Check sheet for the drawn part. Datum: minimum x, y, z corner. Units: mm. A direction names the side the tool comes from. Round coordinates to 2 decimals unless told otherwise and drop trailing zeros. Write each loop counter-clockwise with the first axis right and the second up, starting at its lowest first coordinate (ties: lowest second). Pieces come first, ordered by that corner, then holes. Notation, with made-up numbers: M 79,-18 L 106,-18 A17 ccw 106,10 Z; hole C -7,60.5 d4. An arc over 180 degrees is marked long. One line per item, written item: value. Start each with the question number.
1. Section check D-D (x = 6). Record the boundary of the cut face in (y, z), and give its area (3 significant figures).
2. Access from +Z, -Z, +X, -X, +Y, -Y to the whole of each face (thin tool, end or side, straight path). Record for the marked faces 1 and 2.
3. Section check A-A (x = 4). Record the boundary of the cut face in (y, z).
4. Section check B-B (y = 7.5). Record the boundary of the cut face in (x, z).
5. Scan lines: probe 1 along Z at (x, y) = (6.25, 11.5); probe 2 along Z at (x, y) = (4.75, 9.5); probe 3 along X at (y, z) = (8.25, 18). Record each from-to range of solid material in increasing order. Write a range as [from, to].
6. Section check C-C (z = 20.75). Record the boundary of the cut face in (x, y), and give its area (3 significant figures).
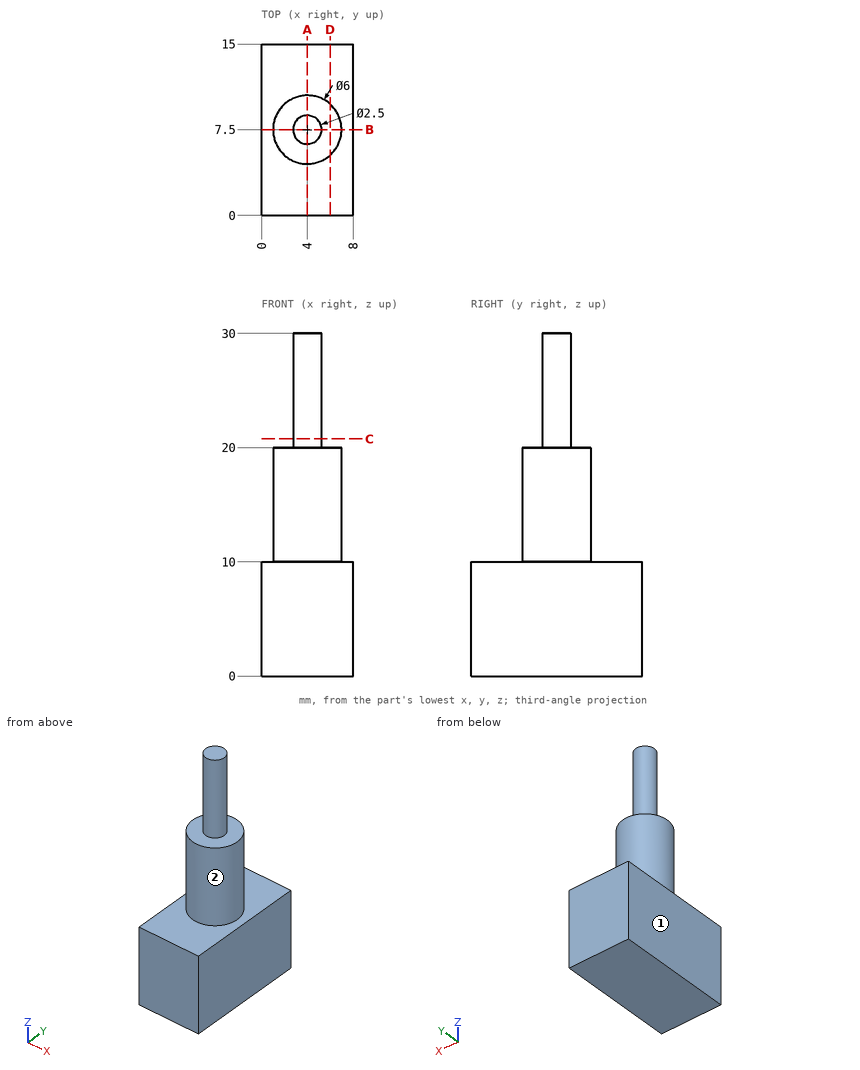
Result sheet:
1. outline: M 0,0 L 15,0 L 15,10 L 9.74,10 L 9.74,20 L 5.26,20 L 5.26,10 L 0,10 Z
1. area: 195 mm2
2. face 1: +Z, -Z, -X, +Y, -Y
2. face 2: +Z
3. outline: M 0,0 L 15,0 L 15,10 L 10.5,10 L 10.5,20 L 8.75,20 L 8.75,30 L 6.25,30 L 6.25,20 L 4.5,20 L 4.5,10 L 0,10 Z
4. outline: M 0,0 L 8,0 L 8,10 L 7,10 L 7,20 L 5.25,20 L 5.25,30 L 2.75,30 L 2.75,20 L 1,20 L 1,10 L 0,10 Z
5. probe 1: z = [0, 10]
5. probe 2: z = [0, 20]
5. probe 3: x = [1.1, 6.9]
6. outline: C 4,7.5 d2.5
6. area: 4.91 mm2
